Build history of the part. All positions in model axes, mm. A direction names the side the tool comes from. Give positions to 0.01 mm unless a question says otherwise; leave off trailing zeros. Order: outer loops, then holes, each group sorted by start corner. A loop starts at its lowest first (then second) coordinate and runs counter-clockwise, first axis right, second up. Notation, with made-up numbers: (85.5, -4.5) -> (139.5, -4.5) arc R12 ccw to (139.5, 6.5) -> close; hole circle Ø1 at (1.5, -30). An arc over 180 degrees is marked (long way). Write item = value, one per line. Start each with the question number.
from build123d import *

# Parameters (mm, degrees)
SKETCH1_R                          = 22.5
EXTRUDE1_DEPTH                     = 8
F_7_X_45_GR_SK_RPNING_VENSTRE_SIZE = 7


with BuildPart() as part:
    # Sketch1 → Extrude1 (new body)
    with BuildSketch(Plane.XY):
        with BuildLine():
            Line((-317, -72.5), (-56.803847577, -72.5))
            ThreePointArc((-56.803847577, -72.5), (-56.027390442, -72.602222521), (-55.303847577, -72.901923789))
            Line((-55.303847577, -72.901923789), (-5.600653599, -101.598076211))
            ThreePointArc((-5.600653599, -101.598076211), (-3.570421982, -101.952770637), (-1.790438983, -100.913872625))
            Line((-1.790438983, -100.913872625), (48.51450695, -40.191325127))
            ThreePointArc((48.51450695, -40.191325127), (62.999688566, 0.19809232), (48.260799916, 40.49561941))
            Line((48.260799916, 40.49561941), (-179.677830313, 312.142300877))
            ThreePointArc((-179.677830313, 312.142300877), (-183.400539462, 314.629735606), (-187.876738219, 314.72740661))
            Line((-187.876738219, 314.72740661), (-194.064678331, 313.069353055))
            ThreePointArc((-194.064678331, 313.069353055), (-196.639749615, 311.854870591), (-198.62642655, 309.815489672))
            Line((-198.62642655, 309.815489672), (-326.192869732, 120.690460119))
            ThreePointArc((-326.192869732, 120.690460119), (-343.285304783, 65.643823322), (-327.156169271, 10.30726627))
            Line((-327.156169271, 10.30726627), (-303.226588641, -26.54105654))
            ThreePointArc((-303.226588641, -26.54105654), (-300.774766081, -42.946584357), (-311.547634765, -55.559992981))
            Line((-311.547634765, -55.559992981), (-318.267854785, -58.693683041))
            ThreePointArc((-318.267854785, -58.693683041), (-319.530174337, -59.800707577), (-320, -61.412606402))
            Line((-320, -61.412606402), (-320, -69.5))
            ThreePointArc((-320, -69.5), (-319.121320344, -71.621320344), (-317, -72.5))
        make_face()
        Circle(SKETCH1_R, mode=Mode.SUBTRACT)
        with BuildLine():
            Line((-193.85365949, 232.607111101), (-178.838777944, 60.98622971))
            ThreePointArc((-178.838777944, 60.98622971), (-191.798712106, 27.885082811), (-225.99409877, 18.173164851))
            ThreePointArc((-225.99409877, 18.173164851), (-284.038197126, 63.350786049), (-280.661065267, 136.826835149))
            Line((-280.661065267, 136.826835149), (-221.786961018, 238.79977496))
            ThreePointArc((-221.786961018, 238.79977496), (-205.549985752, 245.944215066), (-193.85365949, 232.607111101))
        make_face(mode=Mode.SUBTRACT)
    extrude(amount=EXTRUDE1_DEPTH)

    # 7 x 45 gr skærpning - Venstre
    # the kernel refuses this chamfer: 7 mm, written as the material it takes off along each edge
    with BuildSketch(Plane(origin=(-55.303847577, -72.901923789, 8), x_dir=(-0.013747938305292761, -0.02381212764408935, -0.9996219169112969), z_dir=(0.8660254037844379, -0.5000000000000012, 0))) as f_7_x_45_gr_sk_rpning_venstre_piece_1:
        Polygon((F_7_X_45_GR_SK_RPNING_VENSTRE_SIZE * 0.999621916911, F_7_X_45_GR_SK_RPNING_VENSTRE_SIZE * 0.0274958766106), (-F_7_X_45_GR_SK_RPNING_VENSTRE_SIZE * 0.0274958766106, F_7_X_45_GR_SK_RPNING_VENSTRE_SIZE * 0.999621916911), (0, 0), align=None)
    extrude(amount=75.394085761, mode=Mode.SUBTRACT)
    with BuildSketch(Plane(origin=(-56.803847577, -75.5, 8), x_dir=(0, 1, 0), z_dir=(-1, 0, 0))) as f_7_x_45_gr_sk_rpning_venstre_piece_2:
        Polygon((3, F_7_X_45_GR_SK_RPNING_VENSTRE_SIZE), (3 + F_7_X_45_GR_SK_RPNING_VENSTRE_SIZE, 0), (3, 0), align=None)
    revolve(axis=Axis((-56.803847577, -75.5, 8), (0, 0, -1)), revolution_arc=30, mode=Mode.SUBTRACT)
    with BuildSketch(Plane(origin=(-335.001780916, -72.5, 8), x_dir=(0, -0.02749587661058612, -0.9996219169112968), z_dir=(1, 0, 0))) as f_7_x_45_gr_sk_rpning_venstre_piece_3:
        Polygon((F_7_X_45_GR_SK_RPNING_VENSTRE_SIZE * 0.999621916911, F_7_X_45_GR_SK_RPNING_VENSTRE_SIZE * 0.0274958766106), (-F_7_X_45_GR_SK_RPNING_VENSTRE_SIZE * 0.0274958766106, F_7_X_45_GR_SK_RPNING_VENSTRE_SIZE * 0.999621916911), (0, 0), align=None)
    extrude(amount=278.197933338, mode=Mode.SUBTRACT)


solid = part.part
(1) Wall check: line 1 (X direction, y = 186, z = 7.5); line 2 (Y direction, x = 0, z = 3.5); line 3 (Y direction, x = -206, z = 1.25). Give the ranges that are in metal, low to high. Write a range as [from, to].
(2) 3-axis set-ups, long thin cutter, end or side, ignore diameter. For faces 5 (the face through (-205.81, 246, 3.94)), 6 (the face through (-315.36, -7.86, 3.94)), 7 (the face through (-143, 66, 8)): which of +Z, -Z, +X, -X, +Y, -Y reach the whole face in a straight line?
(3) Cut at D-D, the plane y = 214. Give the cut face in (x, z).
(4) Cut at C-C, the plane z = 6.5. Give the cut face in (x, y), plus the area to 3 significant figures.
(5) Cut at A-A, the plane y = 0. Give the cut face in (x, z), plus the area to 3 significant figures.
(6) Cut at B-B, the plane x = -216. Give the cut face in (y, z).
(7) Flat gauge pins, fed straight in: P1, Ø1.5, axis at x = -265, z = 2, coming from the -Y side; P2, Ø0.8, axis at x = -218, z = 0.5, coming from the -Y side; P3, Ø2.5, axis at y = -66.5, z = 2.5, coming from the -X side. Where does each tip first touch, or does it go through?
(8) Mould opens along X. For faces 1 (the face through (-30.8, -87.05, 0.49)), 2 (the face through (-283.584, 62.382, 3.944)), 3 (the face through (-143, 63, 0)), 4 (the face through (63, 0, 4)) say: released by +X, released by -X, zero draft, split by the parting line, or undercut.
Results:
q1.line_1 = [-282.14, -252.27], [-189.78, -73.83]
q1.line_2 = [-98.75, -22.5], [22.5, 98.01]
q1.line_3 = [-72.25, 19.57], [246.04, 298.88]
q2.face_5 = +Z, -Z
q2.face_6 = +Z, -Z, -X
q2.face_7 = +Z, +X, -X, +Y, -Y
q3.outline = (-263.25, 0) -> (-236.11, 0) -> (-236.11, 8) -> (-263.25, 8) -> close; (-192.23, 0) -> (-97.33, 0) -> (-97.33, 8) -> (-192.23, 8) -> close
q4.outline = (-327.16, 10.31) -> (-303.23, -26.54) arc R20 cw to (-311.55, -55.56) -> (-318.27, -58.69) arc R3 ccw to (-320, -61.41) -> (-320, -67) -> (-56.8, -67) arc R8.5 cw to (-52.55, -68.14) -> (0.15, -98.57) -> (48.51, -40.19) arc R63 ccw to (48.26, 40.5) -> (-179.68, 312.14) arc R8 ccw to (-187.88, 314.73) -> (-194.06, 313.07) arc R8 ccw to (-198.63, 309.82) -> (-326.19, 120.69) arc R100 ccw to start; hole (-280.66, 136.83) arc R80 ccw to (-225.99, 18.17) arc R40 ccw to (-178.84, 60.99) -> (-193.85, 232.61) arc R15 ccw to (-221.79, 238.8) -> close; hole circle Ø45 at (0, 0)
q4.area = 81,200 mm2
q5.outline = (-320.46, 0) -> (-22.5, 0) -> (-22.5, 8) -> (-320.46, 8) -> close; (22.5, 0) -> (63, 0) -> (63, 8) -> (22.5, 8) -> close
q5.area = 2,710 mm2
q6.outline = (-72.5, 0) -> (17.59, 0) -> (17.59, 8) -> (-65.5, 8) -> (-72.5, 1) -> close; (244.46, 0) -> (284.06, 0) -> (284.06, 8) -> (244.46, 8) -> close
q7.P1 = -72.25
q7.P2 = -72.5
q7.P3 = -320
q8.face_1 = released by -X
q8.face_2 = undercut
q8.face_3 = zero draft
q8.face_4 = released by +X
